Read the model definition and answer for the solid it produces. Units are mm, in the model's axes. A direction names the side the tool comes from. Give positions to 0.01 mm unless a question says otherwise; leave off trailing zeros. Order: outer loops, then holes, each group sorted by start corner. A loop starts at its lowest first (then second) coordinate and runs counter-clockwise, first axis right, second up. Notation, with made-up numbers: M -31,-14.75 L 18,-14.75 A24 cw 18,14.25 Z; hole C 22.25,10 d3. An arc over 180 degrees is marked long. One line per item, written item: value.
from build123d import *

# Parameters (mm, degrees)
F0_W      = 16
F0_H      = 16
F1_DEPTH  = 16
F2_R      = 3
F3_DEPTH  = 25
F2_R_2    = 5
F4_DEPTH  = 28
F5_R      = 4
F6_DEPTH  = 25
F5_R_2    = 7
F7_DEPTH  = 16
F8_R      = 3
F9_DEPTH  = 16
F8_R_2    = 7
F10_DEPTH = 10


with BuildPart() as f1:
    # F0 (on Top) → F1 (new body)
    with BuildSketch(Plane.XY):
        Rectangle(F0_W, F0_H)
    extrude(amount=F1_DEPTH)

    # F2 (on face) → F3 (cut)
    with BuildSketch(Plane.YZ.offset(8)):
        with Locations((0, 8)):
            Circle(F2_R)
    extrude(amount=-F3_DEPTH, mode=Mode.SUBTRACT)

    # F2 (on face) → F4 (join)
    with BuildSketch(Plane.YZ.offset(8)):
        with Locations((0, 8)):
            Circle(F2_R_2)
        with Locations((0, 8)):
            Circle(F2_R, mode=Mode.SUBTRACT)
    extrude(amount=F4_DEPTH)

    # F5 (on face) → F6 (cut)
    with BuildSketch(Plane.XY.offset(16)):
        Circle(F5_R)
    extrude(amount=-F6_DEPTH, mode=Mode.SUBTRACT)

    # F5 (on face) → F7 (join)
    with BuildSketch(Plane.XY.offset(16)):
        Circle(F5_R_2)
        Circle(F5_R, mode=Mode.SUBTRACT)
    extrude(amount=F7_DEPTH)

    # F8 (on face) → F9 (join)
    with BuildSketch(Plane(origin=(0, 8, 0), x_dir=(-1, 0, 0), z_dir=(0, 1, 0))):
        with Locations((0, 8)):
            Circle(F8_R)
    extrude(amount=F9_DEPTH)

    # F8 (on face) → F10 (join)
    with BuildSketch(Plane(origin=(0, 8, 0), x_dir=(-1, 0, 0), z_dir=(0, 1, 0))):
        with Locations((0, 8)):
            Circle(F8_R_2)
        with Locations((0, 8)):
            Circle(F8_R, mode=Mode.SUBTRACT)
    extrude(amount=F10_DEPTH)


solid = f1.part
1) Consider probe 1 along Z at (x, y) = (4.8, 0); probe 2 along Y at (x, z) = (0, 4.75); probe 3 along Y at (x, z) = (-4.4, 8). Determine where each line is inside the solid, lowest interval first.
Reported:
probe 1: z = 0 to 5, 11 to 32
probe 2: y = -8 to -4, 4 to 18
probe 3: y = -8 to -3, 3 to 18
2) Find section D-D, the plane z = 24. Write down the section's boundary in (x, y), plus the area to 3 significant figures.
Reported:
outline: C 0,0 d14; hole C 0,0 d8
area: 104 mm^2
3) Find section A-A, the plane y = 0. Write down the section's boundary in (x, z).
Reported:
outline: M -8,0 L -4,0 L -4,5 L -8,5 Z; M -8,11 L -4,11 L -4,32 L -7,32 L -7,16 L -8,16 Z; M 4,0 L 8,0 L 8,3 L 36,3 L 36,5 L 4,5 Z; M 4,11 L 36,11 L 36,13 L 8,13 L 8,16 L 7,16 L 7,32 L 4,32 Z
4) Each of these flat-tipped pins is pushed along its axis until it touches: pin 1 Ø3.5 at (y, z) = (0, 8) entering from -X; pin 2 Ø4 at (y, z) = (19, 11.5) entering from +X; pin 3 Ø3 at (x, y) = (-2.5, 15) entering from -Z; pin 4 Ø2 at (x, z) = (5.5, 22.5) entering from +Y. Where does it stop, or does it pass through?
Reported:
pin 1: passes through
pin 2: stops at x = 6.77
pin 3: stops at z = 1.07
pin 4: stops at y = 5.36
5) Find section B-B, the plane z = 8. Write down the section's boundary in (x, y).
Reported:
outline: M -8,-8 L 8,-8 L 8,-5 L 36,-5 L 36,-3 L 2.65,-3 A4 cw -2.65,-3 L -8,-3 Z; M -8,3 L -2.65,3 A4 cw 2.65,3 L 36,3 L 36,5 L 8,5 L 8,8 L 7,8 L 7,18 L 3,18 L 3,24 L -3,24 L -3,18 L -7,18 L -7,8 L -8,8 Z
6) Which of the six approach directions +Z, -Z, +X, -X, +Y, -Y give full straight-line access (tool end or side, diameter ignored) to faces 1 (the face through (3, -3, 32)), 2 (the face through (-7.2, 8, 7.9)), 3 (the face through (8, -4, 4)), 4 (the face through (6.466, -2.681, 23.888))?
Reported:
face 1: +Z, +X, -X, +Y, -Y
face 2: +Y
face 3: +X
face 4: +Z
7) Find section C-C, the plane x = 0. Write down the section's boundary in (y, z), plus the area to 3 significant figures.
Reported:
outline: M -8,0 L -4,0 L -4,32 L -7,32 L -7,16 L -8,16 Z; M 4,0 L 8,0 L 8,1 L 18,1 L 18,5 L 24,5 L 24,11 L 18,11 L 18,15 L 8,15 L 8,16 L 7,16 L 7,32 L 4,32 Z
area: 400 mm^2
